Read the model definition and answer for the solid it produces. Units are mm, in the model's axes. A direction names the side the tool comes from. Round coordinates to 2 decimals unless told otherwise and drop trailing zeros. Write each loop counter-clockwise with the first axis right and the second up, starting at its lowest first coordinate (ties: lowest second). Pieces come first, ordered by that corner, then holes. Notation, with made-up numbers: (59.25, 32.5) - (101.25, 32.5) arc R24 cw to (101.25, 43.5) - close; hole circle Ø6 at (59, 28). An arc over 180 degrees is marked (long way). Use one line per item in the form item = value. Start each with the question number.
1) The part is cut by section D-D, the plane z = -6.5. Give the vertices of the cut face in (x, y) (3 decimals).
2) Each of these flat-tipped pins is pushed along its axis until it touches: pin 1 (6 mm diameter, centred on y = 9.5, z = 1.5, fed in from -X) (3 decimals); pin 2 (2.5 mm diameter, centred on x = -1, y = -1, fed in from +Z); pin 3 (1.6 mm diameter, centred on x = -1, y = -1, fed in from -Z) (3 decimals). Where does it stop, or does it pass through?
3) For faces 4 (the face through (142.875, 3, -3)), 5 (the face through (154.09, 12.93, 4.07)), 6 (the face through (-2, 0, -3.175)), determine the directions among +Z, -Z, +X, -X, +Y, -Y from which every point of the face is accessible in a straight line to the end or side of a thin tool.
4) The part is cut by section A-A, the plane z = 0. Give the vertices of the cut face in (x, y) (3 decimals).
5) For a pull along X with two mould halves and no side action, classify faces 1 (the face through (-15.875, 0, 0)), 2 (the face through (70.87, -0.52, 3.93)), 3 (the face through (-2, 0, 3.175)) as released by +X, released by -X, zero draft, split by the parting line, or undercut.
6) The part is cut by section C-C, the plane x = 90.5. Give the vertices of the cut face in (y, z), plus the area to 3 significant figures.
7) Consider line 1 along X through (y, z) = (-8.5, 6.5) (3 decimals); line 2 along Z through (x, y) = (125.5, 0); line 3 along Y through (x, z) = (75.5, -3.25). Determine where each line is inside the solid, lowest interval first. Write a range as from..to.
8) The part is cut by section B-B, the plane y = 0. Give the vertices of the cut face in (x, z) (3 decimals), plus the area to 3 significant figures.
Autodesk Inventor part; units mm, degrees
ref_plane "dia1_XY" through (-3.175, 3.9624, 0) normal (1, 0, 0) x (0, 0, -1)
ref_plane "dia1_YZ" through (-3.175, 3.9624, 0) normal (0, 0, -1) x (0, 1, 0)
ref_plane "dia1_ZX" through (-3.175, 3.9624, 0) normal (0, 1, 0) x (1, 0, 0)
sketch "Sketch_1" plane through (0, 0, 0) normal (0, 0, 1) x (1, 0, 0)
  line L0 (164.9984, 0) -> (-3.175, 0)
  line L1 (-3.175, 0) -> (-3.175, 3.9624)
  line L2 (-3.175, 3.9624) -> (142.875, 3.9624)
  line L3 (142.875, 3.9624) -> (142.875, 13.5572)
  line L4 (142.875, 13.5572) -> (164.9984, 13.5572)
  line L5 (164.9984, 13.5572) -> (164.9984, 0)
  line L6 (164.9984, 0) -> (-3.175, 0)
revolve "Revolution1" add sketch "Sketch_1" angle 360 about axis through (164.9984, 0, 0) along (1, 0, 0)
sketch "Sketch_3" plane through (0, 0, 0) normal (0, 0, 1) x (1, 0, 0)
  line L0 (-3.175, 0) -> (-15.875, 0)
  line L1 (-15.875, 0) -> (-15.875, 3.3388)
  line L2 (-15.875, 3.3388) -> (-15.2451, 3.9688)
  line L3 (-15.2451, 3.9688) -> (-3.175, 3.9688)
  line L4 (-3.175, 3.9688) -> (-3.175, 0)
  line L5 (-3.175, 0) -> (-15.875, 0)
revolve "Revolution2" add sketch "Sketch_3" angle 360 about axis through (-3.175, 0, 0) along (1, 0, 0)
thread "Thread1"
sketch "Sketch_10" plane through (-3.175, 0, 0) normal (1, 0, 0) x (0, 0, -1)
  line L0 (-7.9248, -7.9248) -> (7.9248, -7.9248)
  line L1 (7.9248, -7.9248) -> (7.9248, 7.9248)
  line L2 (7.9248, 7.9248) -> (-7.9248, 7.9248)
  line L3 (-7.9248, 7.9248) -> (-7.9248, -7.9248)
  line L4 (-3.175, -3.9624) -> (3.175, -3.9624)
  line L5 (3.175, -3.9624) -> (3.175, 3.9624)
  line L6 (3.175, 3.9624) -> (-3.175, 3.9624)
  line L7 (-3.175, 3.9624) -> (-3.175, -3.9624)
extrude "Extrusion1" cut sketch "Sketch_10" along normal blind 3.175
ref_plane "dia1_XY" through (-3.175, 3.9624, 0) normal (1, 0, 0) x (0, 0, -1)
ref_plane "dia1_YZ" through (-3.175, 3.9624, 0) normal (0, 0, -1) x (0, 1, 0)
ref_plane "dia1_ZX" through (-3.175, 3.9624, 0) normal (0, 1, 0) x (1, 0, 0)
ref_plane "dia12_XY" through (0, 0, 14.1351) normal (1, 0, 0) x (0, 0, -1)
ref_plane "dia12_YZ" through (0, 0, 14.1351) normal (0, 0, -1) x (0, 1, 0)
ref_plane "dia12_ZX" through (0, 0, 14.1351) normal (0, 1, 0) x (1, 0, 0)
ref_plane "dia2_XY" through (-3.175, -3.9624, 0) normal (1, 0, 0) x (0, 0, -1)
ref_plane "dia2_YZ" through (-3.175, -3.9624, 0) normal (0, 0, -1) x (0, 1, 0)
ref_plane "dia2_ZX" through (-3.175, -3.9624, 0) normal (0, 1, 0) x (1, 0, 0)
ref_plane "dia22_XY" through (0, 0, -14.1351) normal (1, 0, 0) x (0, 0, -1)
ref_plane "dia22_YZ" through (0, 0, -14.1351) normal (0, 0, -1) x (0, 1, 0)
ref_plane "dia22_ZX" through (0, 0, -14.1351) normal (0, 1, 0) x (1, 0, 0)
ref_plane "rl1_XY" through (-15.875, 0, 0) normal (1, 0, 0) x (0, 0, -1)
ref_plane "rl1_YZ" through (-15.875, 0, 0) normal (0, 0, -1) x (0, 1, 0)
ref_plane "rl1_ZX" through (-15.875, 0, 0) normal (0, 1, 0) x (1, 0, 0)
ref_plane "rl2_XY" through (-3.175, 0, 0) normal (1, 0, 0) x (0, 0, -1)
ref_plane "rl2_YZ" through (-3.175, 0, 0) normal (0, 0, -1) x (0, 1, 0)
ref_plane "rl2_ZX" through (-3.175, 0, 0) normal (0, 1, 0) x (1, 0, 0)
ref_plane "rod_cp_XY" through (0, 0, 0) normal (1, 0, 0) x (0, 0, -1)
ref_plane "rod_cp_YZ" through (0, 0, 0) normal (0, 0, -1) x (0, 1, 0)
ref_plane "rod_cp_ZX" through (0, 0, 0) normal (0, 1, 0) x (1, 0, 0)
ref_plane "thd1_XY" through (-15.875, 3.9688, 0) normal (1, 0, 0) x (0, 0, -1)
ref_plane "thd1_YZ" through (-15.875, 3.9688, 0) normal (0, 0, -1) x (0, 1, 0)
ref_plane "thd1_ZX" through (-15.875, 3.9688, 0) normal (0, 1, 0) x (1, 0, 0)
ref_plane "thd2_XY" through (-15.875, -3.9688, 0) normal (1, 0, 0) x (0, 0, -1)
ref_plane "thd2_YZ" through (-15.875, -3.9688, 0) normal (0, 0, -1) x (0, 1, 0)
ref_plane "thd2_ZX" through (-15.875, -3.9688, 0) normal (0, 1, 0) x (1, 0, 0)
ref_plane "to_rod_clevis_XY" through (-20.701, 0, 0) normal (1, 0, 0) x (0, 0, -1)
ref_plane "to_rod_clevis_YZ" through (-20.701, 0, 0) normal (0, 0, -1) x (0, 1, 0)
ref_plane "to_rod_clevis_ZX" through (-20.701, 0, 0) normal (0, 1, 0) x (1, 0, 0)
ref_plane "wf1_XY" through (-3.175, 0, 0) normal (1, 0, 0) x (0, 0, -1)
ref_plane "wf1_YZ" through (-3.175, 0, 0) normal (0, 0, -1) x (0, 1, 0)
ref_plane "wf1_ZX" through (-3.175, 0, 0) normal (0, 1, 0) x (1, 0, 0)
ref_plane "wf2_XY" through (0, 0, 0) normal (1, 0, 0) x (0, 0, -1)
ref_plane "wf2_YZ" through (0, 0, 0) normal (0, 0, -1) x (0, 1, 0)
ref_plane "wf2_ZX" through (0, 0, 0) normal (0, 1, 0) x (1, 0, 0)
ref_plane "wfw1_XY" through (-3.175, 0, -3.175) normal (0, 1, 0) x (1, 0, 0)
ref_plane "wfw1_YZ" through (-3.175, 0, -3.175) normal (1, 0, 0) x (0, 0, -1)
ref_plane "wfw1_ZX" through (-3.175, 0, -3.175) normal (0, 0, -1) x (0, 1, 0)
ref_plane "wfw2_XY" through (-3.175, 0, 3.175) normal (0, 1, 0) x (1, 0, 0)
ref_plane "wfw2_YZ" through (-3.175, 0, 3.175) normal (1, 0, 0) x (0, 0, -1)
ref_plane "wfw2_ZX" through (-3.175, 0, 3.175) normal (0, 0, -1) x (0, 1, 0)
properties part number "C-094-DP0000_rod"
Geometry results:
q1.outline = (142.875, -11.897) - (164.998, -11.897) - (164.998, 11.897) - (142.875, 11.897) - close
q2.pin_1 = 142.875
q2.pin_2 = 3.95
q2.pin_3 = -3.175
q3.face_4 = -X
q3.face_5 = +X, -X
q3.face_6 = -Z, +Y, -Y
q4.outline = (-15.875, -3.339) - (-15.245, -3.969) - (-3.175, -3.969) - (-3.175, -3.962) - (142.875, -3.962) - (142.875, -13.557) - (164.998, -13.557) - (164.998, 13.557) - (142.875, 13.557) - (142.875, 3.962) - (-3.175, 3.962) - (-3.175, 3.969) - (-15.245, 3.969) - (-15.875, 3.339) - close
q5.face_1 = released by -X
q5.face_2 = zero draft
q5.face_3 = undercut
q6.outline = circle Ø7.92 at (0, 0)
q6.area = 49.3 mm2
q7.line_1 = 142.875..164.998
q7.line_2 = -3.96..3.96
q7.line_3 = -2.27..2.27
q8.outline = (-15.875, -3.339) - (-15.245, -3.969) - (-3.175, -3.969) - (-3.175, -3.175) - (0, -3.175) - (0, -3.962) - (142.875, -3.962) - (142.875, -13.557) - (164.998, -13.557) - (164.998, 13.557) - (142.875, 13.557) - (142.875, 3.962) - (0, 3.962) - (0, 3.175) - (-3.175, 3.175) - (-3.175, 3.969) - (-15.245, 3.969) - (-15.875, 3.339) - close
q8.area = 1,850 mm2
